```python
from build123d import *

# Parameters (mm, degrees)
SKETCH_1_W                   = 36
SKETCH_1_H                   = 66.7
EXTRUDE_1_DEPTH              = 2
HOLE_WIZARD_M4_2_AT_2_COUNT  = 2
HOLE_WIZARD_M4_2_AT_2_PITCH  = 56.7
HOLE_WIZARD_M4_2_AT_3_COUNT  = 2
HOLE_WIZARD_M4_2_AT_3_PITCH  = 62.376998966
HOLE_WIZARD_M4_2_AT_4_COUNT  = 2
HOLE_WIZARD_M4_2_AT_4_PITCH  = 26
FILLET_1_R                   = 2
HOLE_WIZARD_M3_1_D           = 2.5
HOLE_WIZARD_M3_1_CSINK_D     = 3.05
HOLE_WIZARD_M3_1_CSINK_ANGLE = 90
FILLET_2_R                   = 0.8


with BuildPart() as part:
    # 草图1 → 凸台-拉伸1 (new body)
    with BuildSketch(Plane(origin=(0, 0, 0), x_dir=(1, 0, 0), z_dir=(0, 1, 0))):
        Rectangle(SKETCH_1_W, SKETCH_1_H)
    extrude(amount=EXTRUDE_1_DEPTH)

    # 草图4 → M4 螺纹孔2 (revolve, cut)
    with BuildSketch(Plane(origin=(-13, 2, 28.35), x_dir=(0, 0, 1), z_dir=(1, 0, 0))):
        Polygon((0, 0), (0, 2), (1.65, 2), (1.65, 0.375), (2.025, 0), align=None)
    hole_wizard_m4_2 = revolve(axis=Axis((-13, 8.35, 28.35), (0, -1, 0)), mode=Mode.SUBTRACT)

    # M4 螺纹孔2 at 2: M4 螺纹孔2 ×2
    with Locations(*[(0, 0, -i * HOLE_WIZARD_M4_2_AT_2_PITCH) for i in range(1, HOLE_WIZARD_M4_2_AT_2_COUNT)]):
        add(hole_wizard_m4_2, mode=Mode.SUBTRACT)

    # M4 螺纹孔2 at 3: M4 螺纹孔2 ×2
    with Locations(*[Vector(0.41682030926474145, 0, -0.9089889052042635) * (i * HOLE_WIZARD_M4_2_AT_3_PITCH) for i in range(1, HOLE_WIZARD_M4_2_AT_3_COUNT)]):
        add(hole_wizard_m4_2, mode=Mode.SUBTRACT)

    # M4 螺纹孔2 at 4: M4 螺纹孔2 ×2
    with Locations(*[(i * HOLE_WIZARD_M4_2_AT_4_PITCH, 0, 0) for i in range(1, HOLE_WIZARD_M4_2_AT_4_COUNT)]):
        add(hole_wizard_m4_2, mode=Mode.SUBTRACT)

    # 圆角1
    fillet_1_edges = [part.edges().sort_by_distance(p)[0] for p in [
        (-18, 1, 33.35),
        (-18, 1, -33.35),
    ]]
    fillet(fillet_1_edges, radius=FILLET_1_R)

    # M3 螺纹孔1 (through all)
    with Locations(Plane(origin=(0, 2, 0), x_dir=(1, 0, 0), z_dir=(0, 1, 0))):
        with Locations((14, -4), (14, 4)):
            CounterSinkHole(HOLE_WIZARD_M3_1_D / 2, HOLE_WIZARD_M3_1_CSINK_D / 2, counter_sink_angle=HOLE_WIZARD_M3_1_CSINK_ANGLE)

    # 圆角2
    fillet_2_edges = [part.edges().sort_by_distance(p)[0] for p in [
        (1, 0, 33.35),
        (1, 2, 33.35),
        (-18, 0, 0),
        (1, 0, -33.35),
        (-17.414213562, 0, -32.764213562),
        (-17.414213562, 0, 32.764213562),
        (-18, 2, 0),
        (1, 2, -33.35),
        (-17.414213562, 2, -32.764213562),
        (-17.414213562, 2, 32.764213562),
        (18, 0, 0),
        (18, 1, -33.35),
        (18, 1, 33.35),
        (18, 2, 0),
    ]]
    fillet(fillet_2_edges, radius=FILLET_2_R)


solid = part.part
```
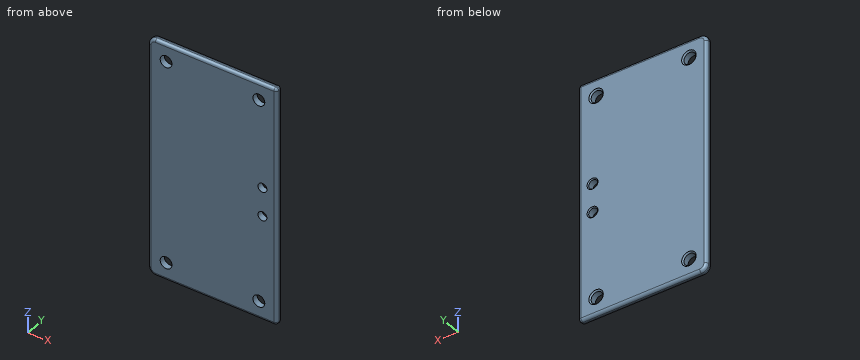
Here's how the part is built. I have some questions about the finished solid (model axes, mm). Coordinates: 2 decimals unless noted, no trailing zeros. Loops run counter-clockwise (first coordinate to the right, second up) from the corner with the lowest first, then second, coordinate; pieces in that order, holes last. Notation, with made-up numbers: (57, -13.5) - (102, -13.5) arc R25 cw to (102, 3.5) - close; hole circle Ø7 at (-32, 5.25). An arc over 180 degrees is marked (long way). Return JSON: item names as keys, results as strings. Group by question number.
Item 1: If we section it at A-A on x = -13: Write out the boundary of the cut face in (y, z) (3 decimals).
Item 2: If we section it at C-C on z = 4: Write out the boundary of the cut face in (x, y) (3 decimals).
Item 3: I need wall thicknesses on line 1 (X direction, y = 0.9, z = -28.35); line 2 (X direction, y = 0.4, z = -28.35); line 3 (Z direction, x = 14, y = 1.3). Which ranges of each line are inside material? Lowest first, please. Write a range as from..to.
Item 4: If we section it at B-B on z = -28.35: Write out the boundary of the cut face in (x, y) (3 decimals), and give its area (3 significant figures).
Item 5: Will these pins go through, and if not, where does the flat tip stop? P1, Ø2.5, axis at x = 13, z = 28.35, coming from the -Y side; P2, Ø4, axis at x = -13, z = -28.35, coming from the +Y side (3 decimals).
Item 6: If we section it at D-D on x = 14: State how many separate pieces and enclosed holes the cut face has, and give its area (3 significant figures).
Calculated:
{
 "1": {"outline": "(0, -32.55) arc R0.8 ccw to (0.8, -33.35) - (1.2, -33.35) arc R0.8 ccw to (2, -32.55) - (2, -30.375) - (1.625, -30) - (0, -30) - close; (0, -26.7) - (1.625, -26.7) - (2, -26.325) - (2, 26.325) - (1.625, 26.7) - (0, 26.7) - close; (0, 30) - (1.625, 30) - (2, 30.375) - (2, 32.55) arc R0.8 ccw to (1.2, 33.35) - (0.8, 33.35) arc R0.8 ccw to (0, 32.55) - close"},
 "2": {"outline": "(-18, 0.8) arc R0.8 ccw to (-17.2, 0) - (12.75, 0) - (12.75, 1.725) - (12.475, 2) - (-17.2, 2) arc R0.8 ccw to (-18, 1.2) - close; (15.25, 0) - (17.2, 0) arc R0.8 ccw to (18, 0.8) - (18, 1.2) arc R0.8 ccw to (17.2, 2) - (15.525, 2) - (15.25, 1.725) - close"},
 "3": {"line 1": "x = -18..-14.65, -11.35..11.35, 14.65..18", "line 2": "x = -17.89..-14.65, -11.35..11.35, 14.65..17.89", "line 3": "z = -33.34..-29.66, -27.04..-5.25, -2.75..2.75, 5.25..27.04, 29.66..33.34"},
 "4": {"outline": "(-18, 0.8) arc R0.8 ccw to (-17.2, 0) - (-14.65, 0) - (-14.65, 1.625) - (-15.025, 2) - (-17.2, 2) arc R0.8 ccw to (-18, 1.2) - close; (-11.35, 0) - (11.35, 0) - (11.35, 1.625) - (10.975, 2) - (-10.975, 2) - (-11.35, 1.625) - close; (14.65, 0) - (17.2, 0) arc R0.8 ccw to (18, 0.8) - (18, 1.2) arc R0.8 ccw to (17.2, 2) - (15.025, 2) - (14.65, 1.625) - close", "area": "58.0 mm^2"},
 "5": {"P1": "passes through", "P2": "stops at y = 1.975"},
 "6": {"separate pieces": "5", "enclosed holes": "0", "area": "112 mm^2"}
}
